Verification items for this drawing (mm, ordinates from the low corner). Round coordinates to 2 decimals unless told otherwise and drop trailing zeros. Order: outer loops, then holes, each group sorted by start corner. A loop starts at its lowest first (then second) coordinate and runs counter-clockwise, first axis right, second up. Notation, with made-up numbers: (15, -10) -> (34, -10) arc R25 ccw to (34, 9) -> close; hole circle Ø2 at (42, 29). An arc over 180 degrees is marked (long way). Use a Markdown table: item, result. Add a question column.
Item 1: Sectioned sample at A-A, the plane z = 5. Record the cut outline in (x, y).
Item 2: Gauge pin test, flat ends, axial feed: pin 1 Ø6 at (y, z) = (3.5, 3) entering from +X; pin 2 Ø2 at (y, z) = (12, 8) entering from +X; pin 3 Ø4.5 at (x, z) = (7.5, 5) entering from -Y; pin 4 Ø6 at (x, z) = (10.5, 4.5) entering from +Y. Record the tip position at first contact, or that the pin passes through.
Item 3: Sectioned sample at B-B, the plane y = 7.5. Record the cut outline in (x, z).
Item 4: Mould release check, pull along X, two halves, no side actions. Record for the marked faces 1, 2, 3 and 4: pulls with the +X half, pulls with the -X half, needs draft (parallel to the pull), parting line crosses it, or undercut.
Item 5: Sectioned sample at D-D, the plane z = 4. Record the cut outline in (x, y), and give its area (3 significant figures).
Item 6: Material ranges on probe 1 along Z at (x, y) = (7.5, 0.95); probe 2 along Y at (x, z) = (1.5, 5); probe 3 along Y at (x, z) = (6.5, 1.75), recorded low to high. Write a range as [from, to].
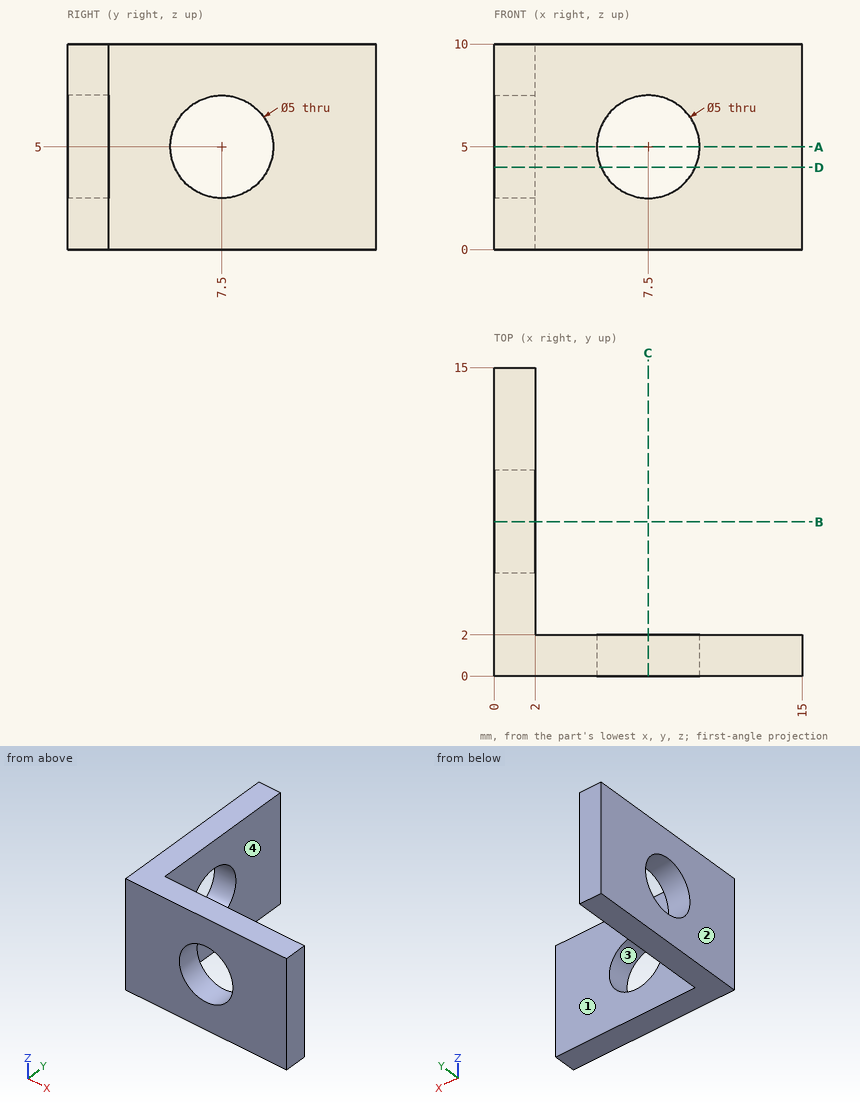
Found:
| question | item | result |
|---|---|---|
| 1 | outline | (0, 0) -> (5, 0) -> (5, 2) -> (2, 2) -> (2, 5) -> (0, 5) -> close; (0, 10) -> (2, 10) -> (2, 15) -> (0, 15) -> close; (10, 0) -> (15, 0) -> (15, 2) -> (10, 2) -> close |
| 2 | pin 1 | stops at x = 15 |
| 2 | pin 2 | stops at x = 2 |
| 2 | pin 3 | passes through |
| 2 | pin 4 | stops at y = 2 |
| 3 | outline | (0, 0) -> (2, 0) -> (2, 2.5) -> (0, 2.5) -> close; (0, 7.5) -> (2, 7.5) -> (2, 10) -> (0, 10) -> close |
| 4 | face 1 | needs draft |
| 4 | face 2 | pulls with the -X half |
| 4 | face 3 | undercut |
| 4 | face 4 | pulls with the +X half |
| 5 | outline | (0, 0) -> (5.21, 0) -> (5.21, 2) -> (2, 2) -> (2, 5.21) -> (0, 5.21) -> close; (0, 9.79) -> (2, 9.79) -> (2, 15) -> (0, 15) -> close; (9.79, 0) -> (15, 0) -> (15, 2) -> (9.79, 2) -> close |
| 5 | area | 37.7 mm2 |
| 6 | probe 1 | z = [0, 2.5], [7.5, 10] |
| 6 | probe 2 | y = [0, 5], [10, 15] |
| 6 | probe 3 | y = [0, 2] |
